Read the model definition and answer for the solid it produces. Units are mm, in the model's axes. A direction names the side the tool comes from. Round coordinates to 2 decimals unless told otherwise and drop trailing zeros. Write each loop counter-clockwise with the first axis right and the second up, starting at its lowest first coordinate (ties: lowest second). Pieces come first, ordered by that corner, then holes.
from build123d import *

# Parameters (mm, degrees)
SKETCH1_R                 = 3
BOSS_EXTRUDE1_DEPTH       = 34.5
SKETCH2_R                 = 5
SKETCH3_R                 = 1
CUT_EXTRUDE1_DEPTH        = 3
DOME1_FACE_RADIUS         = 3
DOME1_HEIGHT              = 0.5
CUT_EXTRUDE2_DEPTH        = 3.5
CIRPATTERN1_COUNT         = 8
FILLET1_R                 = 0.5
CHAMFER1_SIZE             = 0.1
M3X0_5_TAPPED_HOLE1_D     = 2.5
M3X0_5_TAPPED_HOLE1_DEPTH = 6
M3X0_5_TAPPED_HOLE1_TIP   = 0.751075774


with BuildPart() as part:
    # Sketch1 → Boss-Extrude1 (new body)
    with BuildSketch(Plane.XY):
        Circle(SKETCH1_R)
    extrude(amount=-BOSS_EXTRUDE1_DEPTH)

    # Sketch2 → Cut-Revolve1 (revolve, cut)
    with BuildSketch(Plane(origin=(0, 0, 0), x_dir=(0, 0, -1), z_dir=(1, 0, 0)), mode=Mode.PRIVATE) as cut_revolve1_sk:
        with Locations((4, 7.3)):
            Circle(SKETCH2_R)
        Polygon((30, 2.25), (30, 2), (31, 2), (31, 2.25), (34.5, 2.25), (34.5, 3), (28.5, 3), (28.5, 2.25), align=None)
    revolve(cut_revolve1_sk.sketch.rotate(Axis((0, 0, -34.5), (0, 0, 1)), 90), axis=Axis((0, 0, -34.5), (0, 0, 1)), mode=Mode.SUBTRACT)

    # Sketch3 → Cut-Extrude1 (cut, symmetric)
    with BuildSketch(Plane(origin=(0, 0, 0), x_dir=(1, 0, 0), z_dir=(0, 1, 0))):
        with Locations(Location((0, 4, 0), (0, 0, 139.808309089))):
            Circle(SKETCH3_R)
    extrude(amount=CUT_EXTRUDE1_DEPTH, both=True, mode=Mode.SUBTRACT)

    # Dome1: a dome of height H over a round flat face of radius A is a cap of a sphere of radius (A * A + H * H) / (2 * H)
    dome1_r = (DOME1_FACE_RADIUS * DOME1_FACE_RADIUS + DOME1_HEIGHT * DOME1_HEIGHT) / (2 * DOME1_HEIGHT)
    dome1_base = Plane((0, 0, 0), z_dir=(0, 0, 1))
    with Locations(dome1_base.offset(DOME1_HEIGHT - dome1_r)):
        dome1_ball = Sphere(dome1_r, mode=Mode.PRIVATE)
    add(split(dome1_ball, bisect_by=dome1_base, keep=Keep.TOP, mode=Mode.PRIVATE))

    # Sketch4 → Cut-Extrude2 (cut)
    with BuildSketch(Plane(origin=(0, 0, -34.5), x_dir=(-1, 0, 0), z_dir=(0, 0, -1))):
        Polygon((-0.5, 2.5), (-0.318014883, 2), (0.318014883, 2), (0.5, 2.5), align=None)
    cut_extrude2 = extrude(amount=-CUT_EXTRUDE2_DEPTH, mode=Mode.SUBTRACT)

    # CirPattern1: Cut-Extrude2 ×8 about axis
    cirpattern1_axis = Axis((0, 0, 0), (0, 0, 1))
    for i in range(1, CIRPATTERN1_COUNT):
        add(cut_extrude2.rotate(cirpattern1_axis, i * 360 / CIRPATTERN1_COUNT), mode=Mode.SUBTRACT)

    # Fillet1
    fillet1_edges = [part.edges().sort_by_distance(p)[0] for p in [
        (-3, 0, 0),
    ]]
    fillet(fillet1_edges, radius=FILLET1_R)

    # Chamfer1
    chamfer1_edges = [part.edges().sort_by_distance(p)[0] for p in [
        (-3, 0, -28.5),
    ]]
    chamfer(chamfer1_edges, length=CHAMFER1_SIZE)

    # M3x0.5 Tapped Hole1
    with Locations(Plane(origin=(0, 0, -34.5), x_dir=(-1, 0, 0), z_dir=(0, 0, -1))):
        with Locations((0, 0)):
            Hole(M3X0_5_TAPPED_HOLE1_D / 2, depth=M3X0_5_TAPPED_HOLE1_DEPTH)
            with Locations((0, 0, -(M3X0_5_TAPPED_HOLE1_DEPTH + M3X0_5_TAPPED_HOLE1_TIP / 2))):  # 118° drill point
                Cone(0, M3X0_5_TAPPED_HOLE1_D / 2, M3X0_5_TAPPED_HOLE1_TIP, mode=Mode.SUBTRACT)


solid = part.part
Q1. Section C-C (z = -24.5) is taken. Determine the outline of the cut face in (x, y).
Verdict:
outline: circle Ø6 at (0, 0)
Q2. Straight lines are drawn through the part: probe 1 along Y at (x, z) = (0, -31.6); probe 2 along Z at (x, y) = (-0.5, -1.75). For each, find the intervals that lie inside material, in ascending order.
Verdict:
probe 1: y = -2 to -1.25, 1.25 to 2
probe 2: z = -34.5 to -4.87, -3.13 to 0.32
Q3. Section B-B (z = -4) is taken. Determine the outline of the cut face in (x, y), then the cut area to 3 significant figures.
Verdict:
outline: (-1, -2.07) - (-1, 2.07) arc R2.3 ccw to start; (1, -2.07) arc R2.3 ccw to (1, 2.07) - close
area: 7.72 mm2
Q4. Flat-ended cylindrical pins translate along their axes: pin 1 Ø0.9 at (x, y) = (1, -2) entering from +Z; pin 2 Ø2 at (x, y) = (-2, -2) entering from -Z; pin 3 Ø0.6 at (x, y) = (1.5, -0.5) entering from +Z; pin 4 Ø0.5 at (x, z) = (0, -32) entering from -Y. Find the tip coordinate at first contact, or state that the pin passes through.
Verdict:
pin 1: stops at z = 0.33
pin 2: stops at z = -34.5
pin 3: stops at z = 0.41
pin 4: stops at y = -2
Q5. Which of the six approach directions +Z, -Z, +X, -X, +Y, -Y give full straight-line access (tool end or side, diameter ignored) to faces 1 (the cylindrical face through (-2.081, -0.855, -32.774)), 2 (the cylindrical face through (-2.076, 0.867, -32.774)), 3 (the cylindrical face through (2.076, -0.867, -32.774))?
Verdict:
face 1: -Z, -X, -Y
face 2: -Z, -X, +Y
face 3: -Z, +X, -Y
Q6. Determine the mould class of faces 4 (the cylindrical face through (-0.867, -2.076, -32.774)), 5 (the cylindrical face through (-0.27, -1.22, -31.46)), 6 (the cylindrical face through (0.867, 2.076, -32.774)) for opening direction X: pulls with the +X half, pulls with the -X half, needs draft (parallel to the pull), parting line crosses it, or undercut.
Verdict:
face 4: pulls with the -X half
face 5: undercut
face 6: pulls with the +X half
